Drawing for the job (mm, zero at the part's lowest x, y, z). Round coordinates to 2 decimals unless told otherwise and drop trailing zeros. Loops run counter-clockwise (first coordinate to the right, second up) from the corner with the lowest first, then second, coordinate; pieces in that order, holes last.
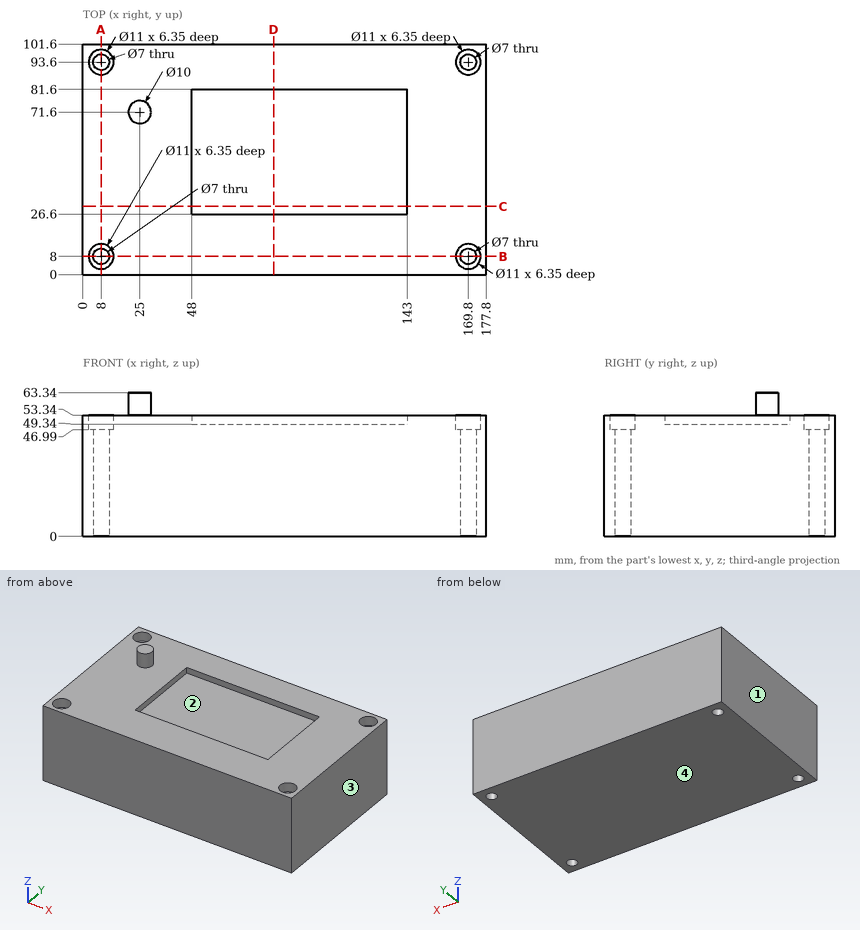
Q1. Flat gauge pins, fed straight in: P1, Ø12, axis at x = 8.5, y = 95.5, coming from the +Z side; P2, Ø10, axis at x = 130, y = 41, coming from the +Z side; P3, Ø5.5, axis at x = 7.5, y = 9, coming from the +Z side. Where does each tip first touch, or does it go through?
Q2. Slice it at D-D on x = 84. Give the cut face in (y, z), plus the area to 3 significant figures.
Q3. Slice it at B-B on y = 8. Give the cut face in (x, z), plus the area to 3 significant figures.
Q4. Pull direction X, two halves, no side cores. Call the marked faces 1, 2, 3 and 4: pulls with the +X half, pulls with the -X half, needs draft (parallel to the pull), parting line crosses it, or undercut.
Q5. Slice it at A-A on x = 8. Give the cut face in (y, z), plus the area to 3 significant figures.
Q6. Probe line 1 (Y direction, x = 8, z = 51); line 2 (Y direction, x = 169, z = 10); line 3 (Z direction, x = 167, y = 54.5). List the from-to ranges inside material, lowest first.
Q7. Slice it at C-C on y = 30. Give the cut face in (x, z), plus the area to 3 significant figures.
Reply:
1. P1: stops at z = 53.34
1. P2: stops at z = 49.34
1. P3: stops at z = 46.99
2. outline: (0, 0) - (101.6, 0) - (101.6, 53.34) - (81.6, 53.34) - (81.6, 49.34) - (26.6, 49.34) - (26.6, 53.34) - (0, 53.34) - close
2. area: 5,200 mm2
3. outline: (0, 0) - (4.5, 0) - (4.5, 46.99) - (2.5, 46.99) - (2.5, 53.34) - (0, 53.34) - close; (11.5, 0) - (166.3, 0) - (166.3, 46.99) - (164.3, 46.99) - (164.3, 53.34) - (13.5, 53.34) - (13.5, 46.99) - (11.5, 46.99) - close; (173.3, 0) - (177.8, 0) - (177.8, 53.34) - (175.3, 53.34) - (175.3, 46.99) - (173.3, 46.99) - close
3. area: 8,690 mm2
4. face 1: pulls with the -X half
4. face 2: undercut
4. face 3: pulls with the +X half
4. face 4: needs draft
5. outline: (0, 0) - (4.5, 0) - (4.5, 46.99) - (2.5, 46.99) - (2.5, 53.34) - (0, 53.34) - close; (11.5, 0) - (90.1, 0) - (90.1, 46.99) - (88.1, 46.99) - (88.1, 53.34) - (13.5, 53.34) - (13.5, 46.99) - (11.5, 46.99) - close; (97.1, 0) - (101.6, 0) - (101.6, 53.34) - (99.1, 53.34) - (99.1, 46.99) - (97.1, 46.99) - close
5. area: 4,620 mm2
6. line 1: y = 0 to 2.5, 13.5 to 88.1, 99.1 to 101.6
6. line 2: y = 0 to 4.59, 11.41 to 90.19, 97.01 to 101.6
6. line 3: z = 0 to 53.34
7. outline: (0, 0) - (177.8, 0) - (177.8, 53.34) - (143, 53.34) - (143, 49.34) - (48, 49.34) - (48, 53.34) - (0, 53.34) - close
7. area: 9,100 mm2
